from build123d import *

# Parameters (mm, degrees)
SKETCH1_R               = 0.5
BOSS_EXTRUDE1_DEPTH     = 5
SKETCH7_R               = 0.75
BOSS_EXTRUDE4_DEPTH     = 0.4
LPATTERN10_COUNT        = 13
LPATTERN10_PITCH        = 0.8
BOSS_EXTRUDE5_DEPTH     = 0.8
CUT_EXTRUDE2_DEPTH      = 8.720265539
CUT_EXTRUDE2_DEPTH_BACK = 8.720265539
SKETCH12_R              = 0.55


with BuildPart() as part:
    # Sketch1 → Boss-Extrude1 (new, symmetric)
    with BuildSketch(Plane(origin=(0, 0, 0), x_dir=(1, 0, 0), z_dir=(0, 1, 0))):
        with Locations(Location((0, 0, 0), (0, 0, 270))):
            Circle(SKETCH1_R)
    extrude(amount=BOSS_EXTRUDE1_DEPTH, both=True)

    # Sketch7 → Boss-Extrude4 (add)
    with BuildSketch(Plane(origin=(0, 5, 0), x_dir=(1, 0, 0), z_dir=(0, 1, 0))):
        with Locations(Location((0, 0, 0), (0, 0, 270))):
            Circle(SKETCH7_R)
    boss_extrude4 = extrude(amount=-BOSS_EXTRUDE4_DEPTH)

    # LPattern10: Boss-Extrude4 ×13
    with Locations(*[(0, -i * LPATTERN10_PITCH, 0) for i in range(1, LPATTERN10_COUNT)]):
        add(boss_extrude4)

    # Sketch10 → Boss-Extrude5 (add, symmetric)
    with BuildSketch(Plane.XY):
        with BuildLine():
            Line((0.75, 5), (-0.85, 5))
            ThreePointArc((-0.85, 5), (-2.05, 6.2), (-0.85, 7.4))
            Line((-0.85, 7.4), (0.75, 7.4))
            Line((0.75, 7.4), (0.75, 5))
        make_face()
    extrude(amount=BOSS_EXTRUDE5_DEPTH, both=True)

    # Sketch12 → Cut-Extrude2 (cut, two sides: drawn at the far end of the back side and taken through both)
    with BuildSketch(Plane.XY.offset(-CUT_EXTRUDE2_DEPTH_BACK)):
        with Locations((-0.85, 6.2)):
            Circle(SKETCH12_R)
    extrude(amount=CUT_EXTRUDE2_DEPTH + CUT_EXTRUDE2_DEPTH_BACK, mode=Mode.SUBTRACT)


solid = part.part
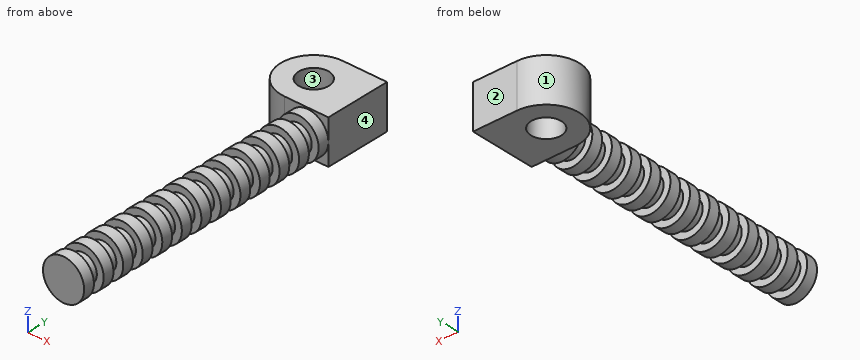
The model under review builds one solid part; all positions refer to its coordinate system, in mm. Face numbers are marked on the shaded views. Round coordinates to 2 decimals unless told otherwise and drop trailing zeros. Loops run counter-clockwise (first coordinate to the right, second up) from the corner with the lowest first, then second, coordinate; pieces in that order, holes last. Notation, with made-up numbers: (56.25, -9) -> (76.25, -9) arc R24 ccw to (76.25, 25) -> close; hole circle Ø8 at (42, 20). An arc over 180 degrees is marked (long way). Answer as CSV lines item,"result".
1) Draft analysis for pull direction X (two halves, no side actions). For the marked faces 1, 2, 3 and 4, state which applies: pulls with the +X half, pulls with the -X half, needs draft (parallel to the pull), parting line crosses it, or undercut.
Geometry results:
face 1,"pulls with the -X half"
face 2,"needs draft"
face 3,"undercut"
face 4,"pulls with the +X half"
2) To check wall thickness, follow line 1 along X through (y, z) = (6.2, 0); line 2 along Y through (x, z) = (-0.85, 0.35); line 3 along Z through (x, y) = (0.05, -3.75). State the ranges of each line that lie inside material, in increasing order. Write a range as from..to.
Geometry results:
line 1,"x = -2.05..-1.4, -0.3..0.75"
line 2,"y = 5..5.65, 6.75..7.4"
line 3,"z = -0.5..0.5"
3) Add section C-C on x = -1.65. Write out the cut boundary in (y, z).
Geometry results:
outline,"(5.31, -0.8) -> (7.09, -0.8) -> (7.09, 0.8) -> (5.31, 0.8) -> close"
4) Add section D-D on y = 2. Write out the cut boundary in (x, z), plus the area to 3 significant figures.
Geometry results:
outline,"circle Ø1 at (0, 0)"
area,"0.785 mm²"
5) Add section B-B on y = 0. Write out the cut boundary in (x, z), plus the area to 3 significant figures.
Geometry results:
outline,"circle Ø1.5 at (0, 0)"
area,"1.77 mm²"
6) Add section A-A on y = 6.2. Write out the cut boundary in (x, z).
Geometry results:
outline,"(-2.05, -0.8) -> (-1.4, -0.8) -> (-1.4, 0.8) -> (-2.05, 0.8) -> close; (-0.3, -0.8) -> (0.75, -0.8) -> (0.75, 0.8) -> (-0.3, 0.8) -> close"
